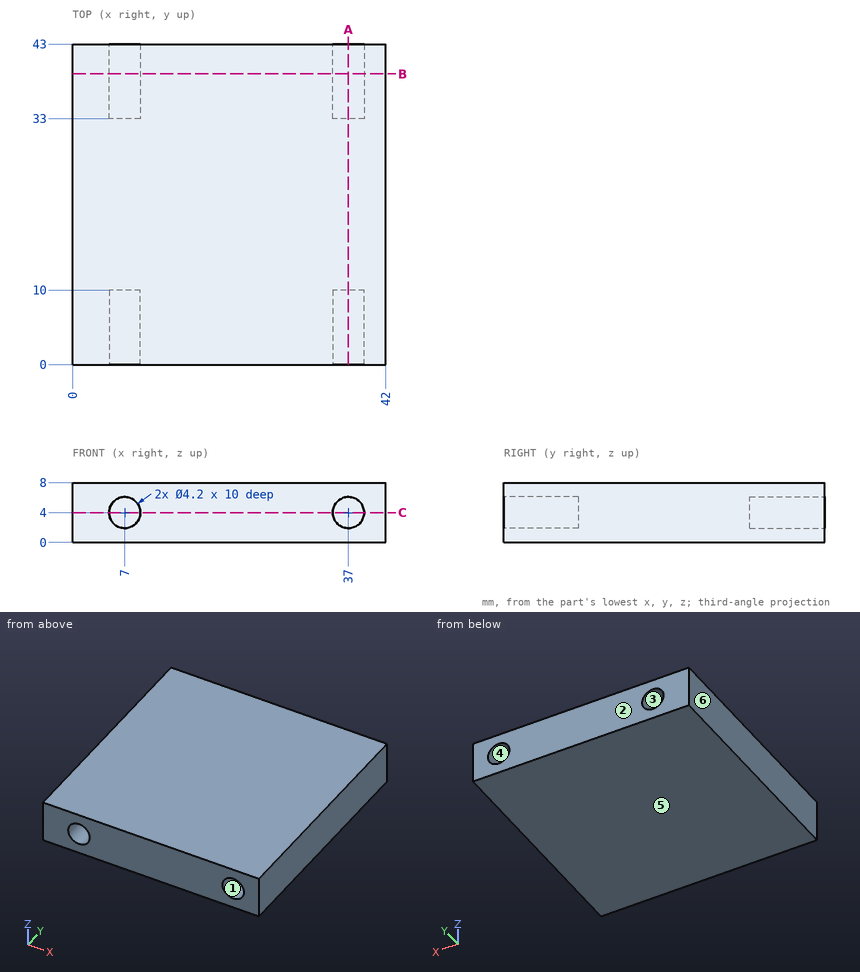
Geometry check sheet. Reference: drawing and pictorial views, mm from the part's lowest x, y, z. A direction names the side the tool comes from. Round coordinates to 2 decimals unless told otherwise and drop trailing zeros. Order: outer loops, then holes, each group sorted by start corner. A loop starts at its lowest first (then second) coordinate and runs counter-clockwise, first axis right, second up. Notation, with made-up numbers: M 50.25,8.25 L 61.25,8.25 A33 ccw 61.25,42.25 Z; hole C 73,63.5 d6. An arc over 180 degrees is marked long. One line per item, written item: value. Start each with the question number.
1. Section check C-C on z = 4. Enter the section's corners in (x, y), and give its area (3 significant figures).
2. Section check B-B on y = 39. Enter the section's corners in (x, z), and give its area (3 significant figures).
3. Access from +Z, -Z, +X, -X, +Y, -Y to the whole of each face (thin tool, end or side, straight path). Record for the marked faces 1, 2 and 3.
4. Section check A-A on x = 37. Enter the section's corners in (y, z).
5. Scan lines: line 1 along X through (y, z) = (39.25, 4); line 2 along Z through (x, y) = (37, 4); line 3 along Y through (x, z) = (37.5, 3.75). Record each from-to range of solid material in increasing order.
6. Release check for a two-part mould opening along X. For the marked faces 4, 5 and 6 record: released by +X, released by -X, zero draft, split by the parting line, or undercut.
7. Gauge pin test, flat ends, axial feed: P1, Ø3.5, axis at x = 7, z = 4, coming from the +Y side; P2, Ø3.5, axis at x = 37, z = 4, coming from the -Y side. Record the tip position at first contact, or that the pin passes through.
Results found:
1. outline: M 0,0 L 4.9,0 L 4.9,10 L 9.1,10 L 9.1,0 L 34.9,0 L 34.9,10 L 39.1,10 L 39.1,0 L 42,0 L 42,43 L 39.1,43 L 39.1,33 L 34.9,33 L 34.9,43 L 9.1,43 L 9.1,33 L 4.9,33 L 4.9,43 L 0,43 Z
1. area: 1,640 mm^2
2. outline: M 0,0 L 42,0 L 42,8 L 0,8 Z; hole C 7,4 d4.2; hole C 37,4 d4.2
2. area: 308 mm^2
3. face 1: -Y
3. face 2: +Z, -Z, +X, -X, +Y
3. face 3: +Y
4. outline: M 0,0 L 43,0 L 43,1.9 L 33,1.9 L 33,6.1 L 43,6.1 L 43,8 L 0,8 L 0,6.1 L 10,6.1 L 10,1.9 L 0,1.9 Z
5. line 1: 0 to 4.9, 9.1 to 34.9, 39.1 to 42
5. line 2: 0 to 1.9, 6.1 to 8
5. line 3: 10 to 33
6. face 4: undercut
6. face 5: zero draft
6. face 6: released by -X
7. P1: y = 33
7. P2: y = 10
